```python
from build123d import *

# Parameters (mm, degrees)
SKETCH_1_W          = 6
SKETCH_1_H          = 40
SKETCH_1_R          = 1.6
SKETCH_1_W_2        = 115
EXTRUDE_1_DEPTH     = 2
CUT_EXTRUDE_1_DEPTH = 2
SKETCH_3_R          = 1.6
CUT_EXTRUDE_2_DEPTH = 67.605179979
CUT_EXTRUDE_3_DEPTH = 67.605179979
CUT_EXTRUDE_4_DEPTH = 67.605179979
SKETCH_6_W          = 35
SKETCH_6_H          = 19
CUT_EXTRUDE_5_DEPTH = 67.605179979


with BuildPart() as part:
    # 草图1 → 凸台-拉伸1 (new body)
    # profile 1 of 3: a face of its own
    with BuildSketch(Plane.XY):
        with Locations((-60.5, 0)):
            Rectangle(SKETCH_1_W, SKETCH_1_H)
        with Locations((-60.5, -5)):
            Circle(SKETCH_1_R, mode=Mode.SUBTRACT)
        with Locations((-60.5, 15)):
            Circle(SKETCH_1_R, mode=Mode.SUBTRACT)
    # profile 2 of 3: a face of its own
    with BuildSketch(Plane.XY):
        Rectangle(SKETCH_1_W_2, SKETCH_1_H)
    # profile 3 of 3: a face of its own
    with BuildSketch(Plane.XY):
        with Locations((60.5, 0)):
            Rectangle(SKETCH_1_W, SKETCH_1_H)
        with Locations((60.5, -5)):
            Circle(SKETCH_1_R, mode=Mode.SUBTRACT)
        with Locations((60.5, 15)):
            Circle(SKETCH_1_R, mode=Mode.SUBTRACT)
    extrude(amount=EXTRUDE_1_DEPTH)

    # 草图2 → 切除-拉伸1 (cut)
    with BuildSketch(Plane.XY.offset(2)):
        with BuildLine():
            Line((3.5, 12), (3.5, -11))
            ThreePointArc((3.5, -11), (0, -14.5), (-3.5, -11))
            Line((-3.5, -11), (-3.5, 12))
            ThreePointArc((-3.5, 12), (0, 15.5), (3.5, 12))
        make_face()
        with BuildLine():
            Line((14, 12), (14, -11))
            ThreePointArc((14, -11), (10.5, -14.5), (7, -11))
            Line((7, -11), (7, 12))
            ThreePointArc((7, 12), (10.5, 15.5), (14, 12))
        make_face()
        with BuildLine():
            Line((24.5, 12), (24.5, -11))
            ThreePointArc((24.5, -11), (21, -14.5), (17.5, -11))
            Line((17.5, -11), (17.5, 12))
            ThreePointArc((17.5, 12), (21, 15.5), (24.5, 12))
        make_face()
        with BuildLine():
            Line((-7, 12), (-7, -11))
            ThreePointArc((-7, -11), (-10.5, -14.5), (-14, -11))
            Line((-14, -11), (-14, 12))
            ThreePointArc((-14, 12), (-10.5, 15.5), (-7, 12))
        make_face()
        with BuildLine():
            Line((-17.5, 12), (-17.5, -11))
            ThreePointArc((-17.5, -11), (-21, -14.5), (-24.5, -11))
            Line((-24.5, -11), (-24.5, 12))
            ThreePointArc((-24.5, 12), (-21, 15.5), (-17.5, 12))
        make_face()
        with BuildLine():
            Line((-28, 12), (-28, -11))
            ThreePointArc((-28, -11), (-31.5, -14.5), (-35, -11))
            Line((-35, -11), (-35, 12))
            ThreePointArc((-35, 12), (-31.5, 15.5), (-28, 12))
        make_face()
        with BuildLine():
            Line((-38.5, 12), (-38.5, -11))
            ThreePointArc((-38.5, -11), (-42, -14.5), (-45.5, -11))
            Line((-45.5, -11), (-45.5, 12))
            ThreePointArc((-45.5, 12), (-42, 15.5), (-38.5, 12))
        make_face()
        with BuildLine():
            Line((-49, 12), (-49, -11))
            ThreePointArc((-49, -11), (-52.5, -14.5), (-56, -11))
            Line((-56, -11), (-56, 12))
            ThreePointArc((-56, 12), (-52.5, 15.5), (-49, 12))
        make_face()
    extrude(amount=-CUT_EXTRUDE_1_DEPTH, mode=Mode.SUBTRACT)

    # 草图3 → 切除-拉伸2 (cut, through all)
    with BuildSketch(Plane.XY.offset(2)):
        with Locations((-48.5, -17)):
            Circle(SKETCH_3_R)
        with Locations((-23.5, -17)):
            Circle(SKETCH_3_R)
        with Locations(Location((23.5, -17, 0), (0, 0, 180))):
            Circle(SKETCH_3_R)
        with Locations(Location((48.5, -17, 0), (0, 0, 180))):
            Circle(SKETCH_3_R)
    extrude(amount=-CUT_EXTRUDE_2_DEPTH, mode=Mode.SUBTRACT)

    # 草图4 → 切除-拉伸3 (cut, through all)
    with BuildSketch(Plane.XY.offset(2)):
        with BuildLine():
            Line((63.5, 5.4), (33.5, 5.4))
            ThreePointArc((33.5, 5.4), (32.5, 4.4), (31.5, 5.4))
            Line((31.5, 5.4), (31.5, 11.4))
            ThreePointArc((31.5, 11.4), (32.5, 12.4), (33.5, 11.4))
            Line((33.5, 11.4), (63.5, 11.4))
            Line((63.5, 11.4), (63.5, 5.4))
        make_face()
    extrude(amount=-CUT_EXTRUDE_3_DEPTH, mode=Mode.SUBTRACT)

    # 草图5 → 切除-拉伸4 (cut, through all)
    with BuildSketch(Plane.XY.offset(2)):
        with BuildLine():
            Line((35, -5), (35, -11))
            ThreePointArc((35, -11), (31.5, -14.5), (28, -11))
            Line((28, -11), (28, -5))
            ThreePointArc((28, -5), (31.5, -1.5), (35, -5))
        make_face()
        with BuildLine():
            Line((45.5, -5), (45.5, -11))
            ThreePointArc((45.5, -11), (42, -14.5), (38.5, -11))
            Line((38.5, -11), (38.5, -5))
            ThreePointArc((38.5, -5), (42, -1.5), (45.5, -5))
        make_face()
        with BuildLine():
            Line((56, -5), (56, -11))
            ThreePointArc((56, -11), (52.5, -14.5), (49, -11))
            Line((49, -11), (49, -5))
            ThreePointArc((49, -5), (52.5, -1.5), (56, -5))
        make_face()
    extrude(amount=-CUT_EXTRUDE_4_DEPTH, mode=Mode.SUBTRACT)

    # 草图6 → 切除-拉伸5 (cut, through all)
    with BuildSketch(Plane.XY.offset(2)):
        with Locations((46, 10.5)):
            Rectangle(SKETCH_6_W, SKETCH_6_H)
    extrude(amount=-CUT_EXTRUDE_5_DEPTH, mode=Mode.SUBTRACT)


solid = part.part
```
The model under review builds one solid part; all positions refer to its coordinate system, in mm. A direction names the side the tool comes from. Round coordinates to 2 decimals unless told otherwise and drop trailing zeros. Loops run counter-clockwise (first coordinate to the right, second up) from the corner with the lowest first, then second, coordinate; pieces in that order, holes last. Notation, with made-up numbers: (88.25, 61) - (92.25, 61) arc R18 ccw to (92.25, 94) - close; hole circle Ø5 at (-13, 28.25). An arc over 180 degrees is marked (long way). Use a Markdown table: item, result. Add a question column.
Q1. Add section C-C (x = -60.5). State the section outline as (y, z) points.
Q2. Machinability: for faces 1 (the face through (-21.1, 15.5, 1)), 2 (the face through (-15, 0, 0)), which of the approach directions +Z, -Z, +X, -X, +Y, -Y give a long, thin tool a straight path to every point of the face, cutting with its end or side? Answer none if there is none.
Q3. For probe 1 along Y at (x, z) = (-60.5, 1.05); probe 2 along Y at (x, z) = (-23.5, 0.75); probe 3 along Y at (x, z) = (48.5, 0.5), list the stretches that pass through material, from the lowest coordinate up.
Q4. The part is to be moulded in two halves that separate along X. For faces 3 (the face through (-18, 20, 1)), 4 (the face through (62.026, -4.519, 0.986)), say which applies: pulls with the +X half, pulls with the -X half, needs draft (parallel to the pull), parting line crosses it, or undercut.
Q5. Add section A-A (y = -17). State the section outline as (x, z) points.
Q6. Insertion check: pin 1 Ø4 at (x, y) = (48.5, -17) entering from +Z; pin 2 Ø1 at (x, z) = (41.5, 1) entering from +Y; pin 3 Ø0.6 at (y, z) = (3.5, 1) entering from +X. Each pin has a flat end and moves straight along its axis. Give the tip position at first contact, or say it passes through.
Q7. Add section D-D (z = 0.8). State how many separate pieces and enclosed holes the cut face has, plus the area to 3 significant figures.
Q8. Add section B-B (x = 60.5). State the section outline as (y, z) points, plus the area to 3 significant figures.
Worked answers:
| question | item | result |
|---|---|---|
| 1 | outline | (-20, 0) - (-6.6, 0) - (-6.6, 2) - (-20, 2) - close; (-3.4, 0) - (13.4, 0) - (13.4, 2) - (-3.4, 2) - close; (16.6, 0) - (20, 0) - (20, 2) - (16.6, 2) - close |
| 2 | face 1 | +Z, -Z |
| 2 | face 2 | -Z, +X, -X, +Y, -Y |
| 3 | probe 1 | -20 to -6.6, -3.4 to 13.4, 16.6 to 20 |
| 3 | probe 2 | -20 to -18.6, -15.4 to -13.45, 14.45 to 20 |
| 3 | probe 3 | -20 to -18.6, -15.4 to 1 |
| 4 | face 3 | needs draft |
| 4 | face 4 | undercut |
| 5 | outline | (-63.5, 0) - (-50.1, 0) - (-50.1, 2) - (-63.5, 2) - close; (-46.9, 0) - (-25.1, 0) - (-25.1, 2) - (-46.9, 2) - close; (-21.9, 0) - (21.9, 0) - (21.9, 2) - (-21.9, 2) - close; (25.1, 0) - (46.9, 0) - (46.9, 2) - (25.1, 2) - close; (50.1, 0) - (63.5, 0) - (63.5, 2) - (50.1, 2) - close |
| 6 | pin 1 | z = 2 |
| 6 | pin 2 | y = 1 |
| 6 | pin 3 | x = 28.5 |
| 7 | separate pieces | 1 |
| 7 | enclosed holes | 18 |
| 7 | area | 2,520 mm² |
| 8 | outline | (-20, 0) - (-6.6, 0) - (-6.6, 2) - (-20, 2) - close; (-3.4, 0) - (1, 0) - (1, 2) - (-3.4, 2) - close |
| 8 | area | 35.6 mm² |
